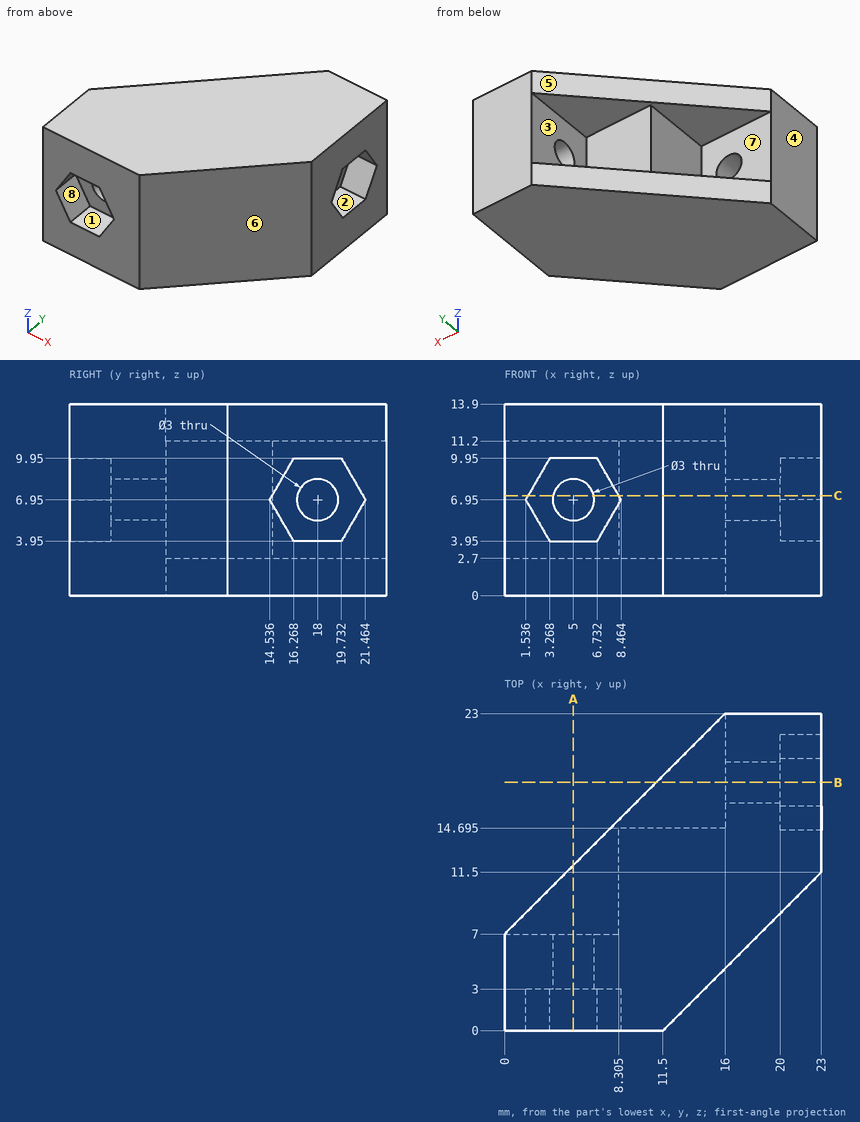
For this review, use the dimensioned drawing (mm, ordinates from the lowest corner) and the shaded views. A direction names the side the tool comes from. Coordinates: 2 decimals unless noted, no trailing zeros. Loops run counter-clockwise (first coordinate to the right, second up) from the corner with the lowest first, then second, coordinate; pieces in that order, holes last. Notation, with made-up numbers: (65, -7) -> (93, -7) arc R29 ccw to (93, 30) -> close; hole circle Ø7 at (71, 55.5). An arc over 180 degrees is marked (long way). Use a Markdown table: item, result. Add a question column.
Item 1: Wall thickness on L1, parallel to Z at x = 5, y = 5; L2, parallel to Z at x = 20.75, y = 17.5; L3, parallel to Y at x = 2.75, z = 4.5: over which ranges is each line inside the solid? List them lowest first. Write a range as from..to.
Item 2: We need section A-A, the plane x = 5. Write out the cut boundary in (y, z).
Item 3: We need section C-C, the plane z = 7.25. Write out the cut boundary in (x, y) (1 decimal), and give its area (3 significant figures).
Item 4: Machinability: for the marked faces 1, 2, 3, 4 and 5, which of the approach directions +Z, -Z, +X, -X, +Y, -Y give a long, thin tool a straight path to every point of the face, cutting with its end or side? Answer none if there is none.
Item 5: We need section B-B, the plane y = 18. Write out the cut boundary in (x, z), and give its area (3 significant figures).
Item 6: Clearance check with flat-ended pins moving along their axes: P1, Ø3, axis at y = 11, z = 2, coming from the -X side; P2, Ø3, axis at x = 5, z = 5.5, coming from the -Y side; P3, Ø8, axis at y = 6.5, z = 12, coming from the +X side; P4, Ø5, axis at y = 17.5, z = 5.5, coming from the +X side. State where each tip first meets the part, or that it passes through.
Item 7: The part is to be moulded in two halves that separate along X. For the marked faces 6, 7 and 8, say which applies: +X half, -X half, draft (parallel to the pull), parting line (faces both ways), or undercut.
Numbers:
| question | item | result |
|---|---|---|
| 1 | L1 | z = 0..5.45, 8.45..13.9 |
| 1 | L2 | z = 0..3.95, 9.95..13.9 |
| 1 | L3 | y = 0..7 |
| 2 | outline | (0, 0) -> (12, 0) -> (12, 2.7) -> (7, 2.7) -> (7, 5.45) -> (3, 5.45) -> (3, 3.95) -> (0, 3.95) -> close; (0, 9.95) -> (3, 9.95) -> (3, 8.45) -> (7, 8.45) -> (7, 11.2) -> (12, 11.2) -> (12, 13.9) -> (0, 13.9) -> close |
| 3 | outline | (0, 0) -> (1.7, 0) -> (1.7, 3) -> (3.5, 3) -> (3.5, 7) -> (0, 7) -> close; (6.5, 3) -> (8.3, 3) -> (8.3, 0) -> (11.5, 0) -> (23, 11.5) -> (23, 14.7) -> (20, 14.7) -> (20, 16.5) -> (16, 16.5) -> (16, 14.7) -> (8.3, 14.7) -> (8.3, 7) -> (6.5, 7) -> close; (16, 19.5) -> (20, 19.5) -> (20, 21.3) -> (23, 21.3) -> (23, 23) -> (16, 23) -> close |
| 3 | area | 203 mm^2 |
| 4 | face 1 | -Y |
| 4 | face 2 | +X |
| 4 | face 3 | -X, +Y |
| 4 | face 4 | +Z, -Z, -X, +Y, -Y |
| 4 | face 5 | +Z, -Z, -X, +Y |
| 5 | outline | (11, 0) -> (23, 0) -> (23, 3.95) -> (20, 3.95) -> (20, 5.45) -> (16, 5.45) -> (16, 2.7) -> (11, 2.7) -> close; (11, 11.2) -> (16, 11.2) -> (16, 8.45) -> (20, 8.45) -> (20, 9.95) -> (23, 9.95) -> (23, 13.9) -> (11, 13.9) -> close |
| 5 | area | 94.3 mm^2 |
| 6 | P1 | stops at x = 2.5 |
| 6 | P2 | stops at y = 3 |
| 6 | P3 | stops at x = 22 |
| 6 | P4 | stops at x = 23 |
| 7 | face 6 | +X half |
| 7 | face 7 | draft |
| 7 | face 8 | undercut |
